```python
from build123d import *

# Parameters (mm, degrees)
SKETCH1_W                                = 80
SKETCH1_H                                = 42
BOSS_EXTRUDE1_DEPTH                      = 8
SKETCH2_W                                = 78
SKETCH2_H                                = 40
CUT_EXTRUDE1_DEPTH                       = 7
FILLET1_R                                = 2
BOSS_EXTRUDE2_REACH                      = 47.88
MIRROR1_AT_THE_SECOND_PLANE_COPY_1_REACH = 47.88
M2_CLEARANCE_HOLE2_D                     = 2.4
SKETCH9_R                                = 2
CUT_EXTRUDE2_DEPTH                       = 2.5
SKETCH11_R                               = 1.25
BOSS_EXTRUDE3_DEPTH                      = 2
FILLET2_R                                = 1
FILLET3_R                                = 1
CUT_EXTRUDE3_REACH                       = 48.271
SKETCH12_R                               = 15


with BuildPart() as part:
    # Sketch1 → Boss-Extrude1 (new body)
    with BuildSketch(Plane(origin=(0, 0, 0), x_dir=(1, 0, 0), z_dir=(0, 1, 0))):
        Rectangle(SKETCH1_W, SKETCH1_H)
    extrude(amount=BOSS_EXTRUDE1_DEPTH)

    # Sketch2 → Cut-Extrude1 (cut)
    with BuildSketch(Plane(origin=(0, 8, 0), x_dir=(1, 0, 0), z_dir=(0, 1, 0))):
        Rectangle(SKETCH2_W, SKETCH2_H)
    extrude(amount=-CUT_EXTRUDE1_DEPTH, mode=Mode.SUBTRACT)

    # Fillet1
    fillet1_edges = [part.edges().sort_by_distance(p)[0] for p in [
        (-39, 4.5, -20),
        (-39, 4.5, 20),
        (39, 4.5, 20),
        (39, 4.5, -20),
        (40, 4, 21),
        (-40, 4, 21),
        (-40, 4, -21),
        (40, 4, -21),
    ]]
    fillet(fillet1_edges, radius=FILLET1_R)

    # Sketch3 → Boss-Extrude2 (add, up to next)
    with BuildSketch(Plane(origin=(0, 8, 0), x_dir=(1, 0, 0), z_dir=(0, 1, 0)), mode=Mode.PRIVATE) as boss_extrude2_sk1:
        with BuildLine():
            Line((-34.5, 18), (-34.5, 20))
            Line((-34.5, 20), (-37, 20))
            ThreePointArc((-37, 20), (-38.414213562, 19.414213562), (-39, 18))
            Line((-39, 18), (-39, 15.5))
            Line((-39, 15.5), (-37, 15.5))
            ThreePointArc((-37, 15.5), (-35.232233047, 16.232233047), (-34.5, 18))
        make_face()
    boss_extrude2_tool1 = extrude(boss_extrude2_sk1.sketch, amount=-BOSS_EXTRUDE2_REACH, mode=Mode.PRIVATE) - part.part
    boss_extrude2 = boss_extrude2_tool1.solids().sort_by_distance((-36.789939, 8, -17.789939))[0]
    add(boss_extrude2)

    # Mirror1: Boss-Extrude2 across plane
    add(boss_extrude2.mirror(Plane.XY))

    # Mirror1 at the second plane: Boss-Extrude2 across plane
    add(boss_extrude2.mirror(Plane(origin=(0, 0, 0), x_dir=(0, 0, 1), z_dir=(1, 0, 0))))

    # Mirror1 at the second plane copy 1 sketc → Mirror1 at the second plane copy 1 (add, up to next)
    with BuildSketch(Plane(origin=(0, 8, 0), x_dir=(-1, 0, 0), z_dir=(0, 1, 0)), mode=Mode.PRIVATE) as mirror1_at_the_second_plane_copy_1_sk1:
        with BuildLine():
            Line((-34.5, 18), (-34.5, 20))
            Line((-34.5, 20), (-37, 20))
            ThreePointArc((-37, 20), (-38.414213562, 19.414213562), (-39, 18))
            Line((-39, 18), (-39, 15.5))
            Line((-39, 15.5), (-37, 15.5))
            ThreePointArc((-37, 15.5), (-35.232233047, 16.232233047), (-34.5, 18))
        make_face()
    mirror1_at_the_second_plane_copy_1_tool1 = extrude(mirror1_at_the_second_plane_copy_1_sk1.sketch, amount=-MIRROR1_AT_THE_SECOND_PLANE_COPY_1_REACH, mode=Mode.PRIVATE) - part.part
    add(mirror1_at_the_second_plane_copy_1_tool1.solids().sort_by_distance((36.789939, 8, 17.789939))[0])

    # M2 Clearance Hole2 (through all)
    with Locations(Plane(origin=(-37, 8, -18), x_dir=(0, 0, 1), z_dir=(0, 1, 0))):
        with Locations((0, 0), (36, 74)):
            Hole(M2_CLEARANCE_HOLE2_D / 2)

    # Sketch9 → Cut-Extrude2 (cut)
    with BuildSketch(Plane.XZ):
        with Locations(Location((-37, -18, 0), (0, 0, 270))):
            Circle(SKETCH9_R)
        with Locations(Location((37, 18, 0), (0, 0, 270))):
            Circle(SKETCH9_R)
    extrude(amount=-CUT_EXTRUDE2_DEPTH, mode=Mode.SUBTRACT)

    # Sketch11 → Boss-Extrude3 (add)
    with BuildSketch(Plane(origin=(0, 8, 0), x_dir=(1, 0, 0), z_dir=(0, 1, 0))):
        with Locations(Location((-37, -18, 0), (0, 0, 90))):
            Circle(SKETCH11_R)
        with Locations(Location((37, 18, 0), (0, 0, 90))):
            Circle(SKETCH11_R)
    extrude(amount=BOSS_EXTRUDE3_DEPTH)

    # Fillet2
    fillet2_edges = [part.edges().sort_by_distance(p)[0] for p in [
        (-37, 10, 19.25),
        (37, 10, -16.75),
    ]]
    fillet(fillet2_edges, radius=FILLET2_R)

    # Fillet3
    fillet3_edges = [part.edges().sort_by_distance(p)[0] for p in [
        (0, 0, -21),
        (40, 0, 0),
        (0, 0, 21),
        (-40, 0, 0),
        (-39.414213562, 0, -20.414213562),
        (-39.414213562, 0, 20.414213562),
        (39.414213562, 0, 20.414213562),
        (39.414213562, 0, -20.414213562),
    ]]
    fillet(fillet3_edges, radius=FILLET3_R - 0.0001)  # a hair under: the kernel refuses the full size

    # Sketch12 → Cut-Extrude3 (cut, up to next)
    with BuildSketch(Plane.XZ, mode=Mode.PRIVATE) as cut_extrude3_sk1:
        with Locations(Location((-10, 0, 0), (0, 0, 270))):
            Circle(SKETCH12_R)
    cut_extrude3_tool1 = extrude(cut_extrude3_sk1.sketch, amount=-CUT_EXTRUDE3_REACH, mode=Mode.PRIVATE) & part.part
    add(cut_extrude3_tool1.solids().sort_by_distance((-10, 0, 0))[0], mode=Mode.SUBTRACT)


solid = part.part
```
Verification items for the finished model (mm, model axes). A direction names the side the tool comes from. Coordinates: 2 decimals unless noted, no trailing zeros. Loops run counter-clockwise (first coordinate to the right, second up) from the corner with the lowest first, then second, coordinate; pieces in that order, holes last. Notation, with made-up numbers: (49, 80.5) -> (100, 80.5) arc R24 ccw to (100, 119.5) -> close; hole circle Ø3 at (7, -20.75). An arc over 180 degrees is marked (long way). Answer in a Markdown table with one row per item. Add a question column.
1. Depth check by flat-ended pin: P1, Ø3, axis at x = 37, z = 18, coming from the +Y side; P2, Ø3.5, axis at x = 37, z = 18, coming from the -Y side; P3, Ø12, axis at x = 2, z = 6, coming from the +Y side. Enter the tip coordinate at first touch or a pass-through.
2. Section check C-C, the plane y = 4. Enter the section's corners in (x, z), then the cut area to 3 significant figures.
3. Section check B-B, the plane x = -10. Enter the section's corners in (y, z), then the cut area to 3 significant figures.
4. Section check A-A, the plane z = 0. Enter the section's corners in (x, y).
5. Access from +Z, -Z, +X, -X, +Y, -Y to the whole of each face (thin tool, end or side, straight path). Record for faces 4 (the face through (38.109, 8.493, -18.577)), 5 (the face through (40, 4, 0)), 6 (the face through (35, 1, 18)).
6. Material ranges on probe 1 along X at (y, z) = (1.35, 18); probe 2 along X at (y, z) = (6.2, -18); probe 3 along X at (y, z) = (2, 9.5), recorded low to high. Write a range as [from, to].
7. Draft check along Z on faces 1 (the face through (-1, 4, -21)), 2 (the face through (39.4, 4.55, 20.43)), 3 (the face through (0, 5, -20)). Enter one of: +Z half, -Z half, draft (parallel to the pull), parting line (faces both ways), or undercut.
Derived:
| question | item | result |
|---|---|---|
| 1 | P1 | stops at y = 8 |
| 1 | P2 | stops at y = 2.5 |
| 1 | P3 | stops at y = 1 |
| 2 | outline | (-40, -19) arc R2 ccw to (-38, -21) -> (38, -21) arc R2 ccw to (40, -19) -> (40, 19) arc R2 ccw to (38, 21) -> (-38, 21) arc R2 ccw to (-40, 19) -> close; hole (-39, -15.5) -> (-37, -15.5) arc R2.5 cw to (-34.5, -18) -> (-34.5, -20) -> (34.5, -20) -> (34.5, -18) arc R2.5 cw to (37, -15.5) -> (39, -15.5) -> (39, 15.5) -> (37, 15.5) arc R2.5 cw to (34.5, 18) -> (34.5, 20) -> (-34.5, 20) -> (-34.5, 18) arc R2.5 cw to (-37, 15.5) -> (-39, 15.5) -> close; hole circle Ø2.4 at (-37, -18); hole circle Ø2.4 at (37, 18) |
| 2 | area | 303 mm² |
| 3 | outline | (0, -20) arc R1 ccw to (1, -21) -> (8, -21) -> (8, -20) -> (1, -20) -> (1, -15) -> (0, -15) -> close; (0, 15) -> (1, 15) -> (1, 20) -> (8, 20) -> (8, 21) -> (1, 21) arc R1 ccw to (0, 20) -> close |
| 3 | area | 25.6 mm² |
| 4 | outline | (-40, 1) arc R1 ccw to (-39, 0) -> (-25, 0) -> (-25, 1) -> (-39, 1) -> (-39, 8) -> (-40, 8) -> close; (5, 0) -> (39, 0) arc R1 ccw to (40, 1) -> (40, 8) -> (39, 8) -> (39, 1) -> (5, 1) -> close |
| 5 | face 4 | +Y |
| 5 | face 5 | +Z, -Z, +X, +Y, -Y |
| 5 | face 6 | -Y |
| 6 | probe 1 | x = [-40, -34.5], [34.5, 35], [39, 40] |
| 6 | probe 2 | x = [-40, -38.2], [-35.8, -34.5], [34.5, 40] |
| 6 | probe 3 | x = [-40, -39], [39, 40] |
| 7 | face 1 | -Z half |
| 7 | face 2 | +Z half |
| 7 | face 3 | undercut |
